```python
from build123d import *

# Parameters (mm, degrees)
BOSS_EXTRUDE1_DEPTH = 4
BOSS_EXTRUDE2_DEPTH = 4


with BuildPart() as part:
    # Sketch1 → Boss-Extrude1 (new body)
    with BuildSketch(Plane.XY):
        Polygon((47, 32.200893004), (54.5, 32.200893004), (54.5, 27.450893004), (62.5, 27.450893004), (62.5, 19.450893004), (54.5, 19.450893004), (54.5, 14.700893004), (47, 14.700893004), (47, -27.799106996), (-81, -27.799106996), (-81, 32.200893004), align=None)
    extrude(amount=BOSS_EXTRUDE1_DEPTH)

    # Sketch2 → Boss-Extrude2 (add)
    with BuildSketch(Plane.XY):
        Polygon((-81, 32.200893004), (54.5, 32.200893004), (54.5, 56.612431949), (39.5, 56.612431949), (25.946325432, 43.058757381), (-51.857864376, 43.058757381), (-66, 57.200893004), (-81, 57.200893004), align=None)
    extrude(amount=BOSS_EXTRUDE2_DEPTH)


solid = part.part
```
The model under review builds one solid part; all positions refer to its coordinate system, in mm. A direction names the side the tool comes from. Give positions to 0.01 mm unless a question says otherwise; leave off trailing zeros. Write each loop counter-clockwise with the first axis right and the second up, starting at its lowest first coordinate (ties: lowest second). Pieces come first, ordered by that corner, then holes.
(1) Tool access review of faces 5 (the flat face through (-10, 15, 4)), 6 (the flat face through (51, 14.701, 2)), 7 (the flat face through (58, 27.451, 2)), 8 (the flat face through (62.5, 24, 2)), 9 (the flat face through (32.82, 49.93, 1.97)): name each direction out of +Z, -Z, +X, -X, +Y, -Y from which nothing blocks a thin tool from reaching the whole face with its end or side.
(2) For P1, Ø2, axis at x = 58.5, z = 1.5, coming from the -Y side; P2, Ø1.2, axis at x = 52.5, z = 2.5, coming from the -Y side; P3, Ø2, axis at y = -13.5, z = 0.5, coming from the +X side, all flat-tipped, find the tip position at first contact; note any pin that passes through.
(3) Consider section C-C, the plane y = 18. Give the boundary of the cut face in (x, z), and give its area (3 significant figures).
(4) To check wall thickness, follow L1, parallel to Y at x = -47.5, z = 2.9; L2, parallel to Y at x = 45, z = 1.35; L3, parallel to X at y = 29.5, z = 0.5. State the ranges of each line that lie inside material, in increasing order.
(5) The part is to be moulded in two halves that separate along X. For faces 1 (the flat face through (-81, 15, 2)), 2 (the flat face through (54.5, 17, 2)), 3 (the flat face through (59, 19.451, 2)), 4 (the flat face through (-12, 43.059, 2)), say which applies: released by +X, released by -X, zero draft, split by the parting line, or undercut.
(6) Consider section B-B, the plane x = 5. Give the boundary of the cut face in (y, z), and give its area (3 significant figures).
(7) Consider section A-A, the plane z = 1.25. Give the boundary of the cut face in (x, y), and give its area (3 significant figures).
Returned:
1. face 5: +Z, +X, -X, +Y, -Y
1. face 6: +Z, -Z, +X, -Y
1. face 7: +Z, -Z, +X, +Y
1. face 8: +Z, -Z, +X, +Y, -Y
1. face 9: +Z, -Z, +Y
2. P1: stops at y = 19.45
2. P2: stops at y = 14.7
2. P3: stops at x = 47
3. outline: (-81, 0) - (54.5, 0) - (54.5, 4) - (-81, 4) - close
3. area: 542 mm2
4. L1: y = -27.8 to 43.06
4. L2: y = -27.8 to 56.61
4. L3: x = -81 to 54.5
5. face 1: released by -X
5. face 2: released by +X
5. face 3: zero draft
5. face 4: undercut
6. outline: (-27.8, 0) - (43.06, 0) - (43.06, 4) - (-27.8, 4) - close
6. area: 283 mm2
7. outline: (-81, -27.8) - (47, -27.8) - (47, 14.7) - (54.5, 14.7) - (54.5, 19.45) - (62.5, 19.45) - (62.5, 27.45) - (54.5, 27.45) - (54.5, 56.61) - (39.5, 56.61) - (25.95, 43.06) - (-51.86, 43.06) - (-66, 57.2) - (-81, 57.2) - close
7. area: 9,950 mm2
